```python
from build123d import *

# Parameters (mm, degrees)
F3_R     = 5
F4_DEPTH = 15
F5_R     = 8.305738
F6_DEPTH = 3
F7_SIZE2 = 2
F7_SIZE  = 0.5


with BuildPart() as f1:
    # F0 (on Top) → F1 (revolve)
    with BuildSketch(Plane.XY):
        with BuildLine():
            ThreePointArc((0, -11.5), (8.131728, -8.131728), (11.5, 0))
            ThreePointArc((11.5, 0), (8.131728, 8.131728), (0, 11.5))
            Line((0, 11.5), (0, -11.5))
        make_face()
    revolve(axis=Axis((0, -5.406174, 0), (0, -1, 0)))

    # F3 (on face) → F4 (cut)
    with BuildSketch(Plane.XZ.offset(11.5)):
        Circle(F3_R)
    extrude(amount=-F4_DEPTH, mode=Mode.SUBTRACT)

    # F5 (on face) → F6 (cut)
    with BuildSketch(Plane.XZ.offset(11.5)):
        Circle(F5_R)
    extrude(amount=-F6_DEPTH, mode=Mode.SUBTRACT)

    # F7
    f7_edges = [f1.edges().sort_by_distance(p)[0] for p in [
        (-5, -8.5, 0),
    ]]
    chamfer(f7_edges, length=F7_SIZE, length2=F7_SIZE2)


solid = f1.part
```
Model file for the job. Use its own axes, mm. Give positions to 0.01 mm unless a question says otherwise; leave off trailing zeros. Write each loop counter-clockwise with the first axis right and the second up, starting at its lowest first coordinate (ties: lowest second). Pieces come first, ordered by that corner, then holes. Notation, with made-up numbers: (44.25, -10.5) -> (93.25, -10.5) arc R11 ccw to (93.25, 4.5) -> close; hole circle Ø7 at (56, 18.25). An arc over 180 degrees is marked (long way). Use CSV: the item, a comma, the result in double quotes. Start each with the question number.
1) Cut at A-A on z = 0. List the corners of the cut face in (x, y), plus the area to 3 significant figures.
2) Cut at B-B on x = 0. List the corners of the cut face in (y, z).
3) Drill centre lines: L1, parallel to Z at x = 0, y = 0.25; L2, parallel to X at y = 7.5, z = 4; L3, parallel to Z at x = 0, y = -4.25. Where is each one in solid material? Low to high.
4) Pin check, flat tips, straight feed: P1, Ø10, axis at y = -5, z = 6, coming from the +X side; P2, Ø5, axis at x = -4, z = -0.5, coming from the +Y side; P3, Ø1, axis at y = 2.5, z = 0.5, coming from the -X side. Stop position of each tip, or through.
5) Two-plate mould, pull along X, no slides. Class faces 1 (the flat face through (3, -8.5, -5)), 2 (the cylindrical face through (-1.08, -1.57, -4.88)), 3 (the flat face through (0, 3.5, 0)): released by +X, released by -X, zero draft, split by the parting line, or undercut.
6) Cut at D-D on y = 8. List the corners of the cut face in (x, z), plus the area to 3 significant figures.
7) Cut at C-C on y = 2. List the corners of the cut face in (x, z).
Final values:
1,outline,"(-7.75, -8.5) -> (-5.5, -8.5) -> (-5, -6.5) -> (-5, 3.5) -> (5, 3.5) -> (5, -6.5) -> (5.5, -8.5) -> (7.75, -8.5) arc R11.5 ccw (long way) to start"
1,area,"263 mm2"
2,outline,"(-8.5, -7.75) arc R11.5 ccw (long way) to (-8.5, 7.75) -> (-8.5, 5.5) -> (-6.5, 5) -> (3.5, 5) -> (3.5, -5) -> (-6.5, -5) -> (-8.5, -5.5) -> close"
3,L1,"z = -11.5 to -5, 5 to 11.5"
3,L2,"x = -7.75 to 7.75"
3,L3,"z = -10.69 to -5, 5 to 10.69"
4,P1,"stops at x = 11.15"
4,P2,"stops at y = 11.4"
4,P3,"stops at x = -11.32"
5,face 1,"zero draft"
5,face 2,"undercut"
5,face 3,"undercut"
6,outline,"circle Ø16.52 at (0, 0)"
6,area,"214 mm2"
7,outline,"circle Ø22.65 at (0, 0); hole circle Ø10 at (0, 0)"
